from build123d import *
from OCP.BRepFilletAPI import BRepFilletAPI_MakeChamfer

# Parameters (mm, degrees)
EXTRUDE_1_DEPTH     = 1
EXTRUDE_2_DEPTH     = 1
SKETCH_3_W          = 1.5
SKETCH_3_H          = 8
EXTRUDE_3_DEPTH     = 4.5
SKETCH_4_W          = 3
SKETCH_4_H          = 1.3
EXTRUDE_4_DEPTH     = 6
FILLET_1_R          = 1
CHAMFER_1_SIZE      = 0.3
SKETCH_5_W          = 5
SKETCH_5_H          = 2
CUT_EXTRUDE_1_DEPTH = 1
SKETCH_6_W          = 4
SKETCH_6_H          = 1
EXTRUDE_5_DEPTH     = 2.3
SKETCH_7_W          = 1.15
SKETCH_7_H          = 4
EXTRUDE_6_DEPTH     = 1
CUT_EXTRUDE_2_REACH = 20.465
SKETCH_10_W         = 4
SKETCH_10_H         = 1.5
FILLET_2_R          = 0.75
SKETCH_11_W         = 1.15
SKETCH_11_H         = 4
EXTRUDE_7_DEPTH     = 1
CHAMFER_2_SIZE      = 1.2
CHAMFER_2_SIZE2     = 1.043144085


with BuildPart() as part:
    # 草图1 → 凸台-拉伸1 (new body)
    with BuildSketch(Plane(origin=(0, 0, 0), x_dir=(0, 0, -1), z_dir=(1, 0, 0))):
        with BuildLine():
            Line((-8.62016793, -6.710374314), (-8.62016793, 4.289625686))
            ThreePointArc((-8.62016793, 4.289625686), (-8.327274711, 4.996732467), (-7.62016793, 5.289625686))
            Line((-7.62016793, 5.289625686), (12.37983207, 5.289625686))
            ThreePointArc((12.37983207, 5.289625686), (13.086938851, 4.996732467), (13.37983207, 4.289625686))
            Line((13.37983207, 4.289625686), (13.37983207, -6.710374314))
            ThreePointArc((13.37983207, -6.710374314), (13.086938851, -7.417481096), (12.37983207, -7.710374314))
            Line((12.37983207, -7.710374314), (-7.62016793, -7.710374314))
            ThreePointArc((-7.62016793, -7.710374314), (-8.327274711, -7.417481096), (-8.62016793, -6.710374314))
        make_face()
    extrude(amount=EXTRUDE_1_DEPTH)

    # 草图2 → 凸台-拉伸2 (add)
    with BuildSketch(Plane.ZY):
        with BuildLine():
            Line((9.62016793, -6.810374314), (9.62016793, 4.189625686))
            ThreePointArc((9.62016793, 4.189625686), (9.063670815, 5.53312857), (7.72016793, 6.089625686))
            Line((7.72016793, 6.089625686), (-12.27983207, 6.089625686))
            ThreePointArc((-12.27983207, 6.089625686), (-13.623334954, 5.53312857), (-14.17983207, 4.189625686))
            Line((-14.17983207, 4.189625686), (-14.17983207, -6.810374314))
            ThreePointArc((-14.17983207, -6.810374314), (-13.623334954, -8.153877199), (-12.27983207, -8.710374314))
            Line((-12.27983207, -8.710374314), (7.72016793, -8.710374314))
            ThreePointArc((7.72016793, -8.710374314), (9.063670815, -8.153877199), (9.62016793, -6.810374314))
        make_face()
    extrude(amount=EXTRUDE_2_DEPTH)

    # 草图3 → 凸台-拉伸3 (add)
    with BuildSketch(Plane(origin=(1, 0, 0), x_dir=(0, 0, -1), z_dir=(1, 0, 0))):
        with Locations((-6.37016793, -1.310374314)):
            Rectangle(SKETCH_3_W, SKETCH_3_H)
        with Locations((10.92983207, -1.310374314)):
            Rectangle(SKETCH_3_W, SKETCH_3_H)
    extrude(amount=EXTRUDE_3_DEPTH)

    # 草图4 → 凸台-拉伸4 (add)
    with BuildSketch(Plane(origin=(1, 0, 0), x_dir=(0, 0, -1), z_dir=(1, 0, 0))):
        with Locations((-5.62016793, -1.999635097)):
            Rectangle(SKETCH_4_W, SKETCH_4_H)
        with Locations((10.17983207, -1.999635097)):
            Rectangle(SKETCH_4_W, SKETCH_4_H)
    extrude(amount=EXTRUDE_4_DEPTH)

    # 圆角1
    fillet_1_edges = [part.edges().sort_by_distance(p)[0] for p in [
        (7, -1.999635097, -8.67983207),
        (7, -1.999635097, -11.67983207),
        (5.5, -5.310374314, 6.37016793),
        (5.5, 2.689625686, 6.37016793),
        (5.5, -5.310374314, -10.92983207),
        (5.5, 2.689625686, -10.92983207),
        (7, -1.999635097, 7.12016793),
        (7, -1.999635097, 4.12016793),
    ]]
    fillet(fillet_1_edges, radius=FILLET_1_R)

    # 倒角1
    chamfer_1_edges = [part.edges().sort_by_distance(p)[0] for p in [
        (5.75, -2.649635097, 7.12016793),
        (5.75, -1.349635097, 7.12016793),
        (5.75, -1.349635097, -11.67983207),
        (5.75, -2.649635097, -11.67983207),
        (7, -2.649635097, -10.17983207),
        (7, -1.349635097, -10.17983207),
        (3.5, -2.649635097, -8.67983207),
        (6.707106781, -2.649635097, -11.386938851),
        (6.707106781, -2.649635097, -8.972725289),
        (3.5, -1.349635097, -8.67983207),
        (6.707106781, -1.349635097, -11.386938851),
        (6.707106781, -1.349635097, -8.972725289),
        (7, -2.649635097, 5.62016793),
        (7, -1.349635097, 5.62016793),
        (3.5, -2.649635097, 4.12016793),
        (6.707106781, -2.649635097, 4.413061149),
        (6.707106781, -2.649635097, 6.827274711),
        (3.5, -1.349635097, 4.12016793),
        (6.707106781, -1.349635097, 4.413061149),
        (6.707106781, -1.349635097, 6.827274711),
    ]]
    chamfer(chamfer_1_edges, length=CHAMFER_1_SIZE)

    # 草图5 → 切除-拉伸1 (cut)
    with BuildSketch(Plane(origin=(1, 0, 0), x_dir=(0, 0, -1), z_dir=(1, 0, 0))):
        with Locations((2.27983207, -6.710374314)):
            Rectangle(SKETCH_5_W, SKETCH_5_H)
        with Locations((2.27983207, 4.289625686)):
            Rectangle(SKETCH_5_W, SKETCH_5_H)
    extrude(amount=-CUT_EXTRUDE_1_DEPTH, mode=Mode.SUBTRACT)

    # 草图6 → 凸台-拉伸5 (add)
    with BuildSketch(Plane(origin=(0, 0, 0), x_dir=(0, 0, -1), z_dir=(1, 0, 0))):
        with Locations((2.27983207, -7.210374314)):
            Rectangle(SKETCH_6_W, SKETCH_6_H)
        with Locations((2.27983207, 4.789625686)):
            Rectangle(SKETCH_6_W, SKETCH_6_H)
    extrude(amount=EXTRUDE_5_DEPTH)

    # 草图7 → 凸台-拉伸6 (add)
    with BuildSketch(Plane.XZ.offset(7.710374314)):
        with Locations((1.725, -2.27983207)):
            Rectangle(SKETCH_7_W, SKETCH_7_H)
    extrude(amount=EXTRUDE_6_DEPTH)

    # 草图10 → 切除-拉伸2 (cut, up to next)
    with BuildSketch(Plane.ZY.offset(1), mode=Mode.PRIVATE) as cut_extrude_2_sk1:
        with Locations((-2.27983207, -4.523813103)):
            Rectangle(SKETCH_10_W, SKETCH_10_H)
    cut_extrude_2_tool1 = extrude(cut_extrude_2_sk1.sketch, amount=-CUT_EXTRUDE_2_REACH, mode=Mode.PRIVATE) & part.part
    add(cut_extrude_2_tool1.solids().sort_by_distance((-1, -4.523813, -2.279832))[0], mode=Mode.SUBTRACT)

    # 圆角2
    fillet_2_edges = [part.edges().sort_by_distance(p)[0] for p in [
        (0, -5.273813103, -0.27983207),
        (0, -3.773813103, -0.27983207),
        (0, -3.773813103, -4.27983207),
        (0, -5.273813103, -4.27983207),
    ]]
    fillet(fillet_2_edges, radius=FILLET_2_R - 0.0001)  # a hair under: the kernel refuses the full size

    # 草图11 → 凸台-拉伸7 (add)
    with BuildSketch(Plane(origin=(0, 5.289625686, 0), x_dir=(1, 0, 0), z_dir=(0, 1, 0))):
        with Locations((1.725, 2.27983207)):
            Rectangle(SKETCH_11_W, SKETCH_11_H)
    extrude(amount=EXTRUDE_7_DEPTH)

    # 倒角2: one chamfer whose edges measure the first distance from different faces: ONE call of the kernel's chamfer builder (chamfer() names one face for all edges)
    chamfer_2_edges_1 = [part.edges().sort_by_distance(p)[0] for p in [
        (2.3, -8.710374314, -2.27983207),
    ]]
    chamfer_2_side_1 = [part.faces().sort_by_distance(p)[0] for p in [
        (2.3, -7.710374314, -2.27983207),
    ]]
    chamfer_2_edges_2 = [part.edges().sort_by_distance(p)[0] for p in [
        (2.3, 6.289625686, -2.27983207),
    ]]
    chamfer_2_side_2 = [part.faces().sort_by_distance(p)[0] for p in [
        (2.3, 5.289625686, -2.27983207),
    ]]
    chamfer_2 = BRepFilletAPI_MakeChamfer(part.part.solid().wrapped)
    for e in chamfer_2_edges_1:
        chamfer_2.Add(CHAMFER_2_SIZE, CHAMFER_2_SIZE2, e.wrapped, chamfer_2_side_1[0].wrapped)  # the first distance lies on this face
    for e in chamfer_2_edges_2:
        chamfer_2.Add(CHAMFER_2_SIZE, CHAMFER_2_SIZE2, e.wrapped, chamfer_2_side_2[0].wrapped)  # the first distance lies on this face
    add(Compound.cast(chamfer_2.Shape()), mode=Mode.REPLACE)


solid = part.part
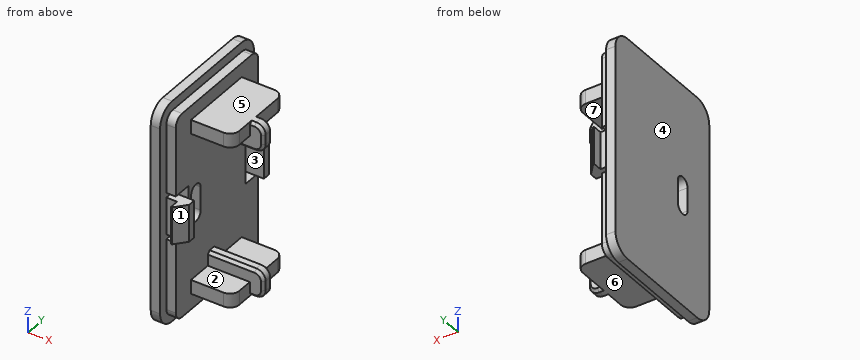
Source: CAD feature listing. Evaluate the final solid. Frame: model axes, mm. Face numbers are marked on the shaded views. A direction names the side the tool comes from. Round coordinates to 2 decimals unless told otherwise and drop trailing zeros. Loops run counter-clockwise (first coordinate to the right, second up) from the corner with the lowest first, then second, coordinate; pieces in that order, holes last. Notation, with made-up numbers: M 56,87 L 69,87 A23 ccw 69,104 Z; hole C 64.25,-30 d11. An arc over 180 degrees is marked long. Return JSON: item names as keys, results as strings. Group by question number.
1. Section query B-B on x = 4. Output: boundary loops of the cut face in (y, z), and give its area (3 significant figures).
2. Section query A-A on z = -2.25. Output: boundary loops of the cut face in (x, y).
3. Mould query, pull axis Y, two halves, no side actions, for the marked faces 1, 2 and 3. Classes: released by +Y, released by -Y, zero draft, split by the parting line, or undercut.
4. Section query D-D on z = 1.25. Output: boundary loops of the cut face in (x, y), and give its area (3 significant figures).
5. Section query C-C on y = -0.5. Output: boundary loops of the cut face in (x, z), and give its area (3 significant figures).
6. Material intervals for line 1 along Z through (x, y) = (3.25, -4.25); line 2 along Y through (x, z) = (4.5, -10); line 3 along X through (y, z) = (5.5, -10.5), sorted ascending. Write a range as from..to.
7. Reachability of the marked faces 4, 5, 6 and 7 from +Z, -Z, +X, -X, +Y, -Y: full face, straight path, thin tool, end or side. Return the list, or none.
8. Pin query (flat end, axial travel): pin 1 (0.8 mm diameter, centred on x = 0.5, z = 5.5, fed in from +Y); pin 2 (1.6 mm diameter, centred on x = 1.5, y = 5.5, fed in from +Z); pin 3 (1.5 mm diameter, centred on x = 4, z = -11, fed in from -Y); pin 4 (1.5 mm diameter, centred on x = 4.5, z = -2, fed in from -Y). Return the tip coordinate at first contact, or that it passes through.
Checks:
{
 "1": {"outline": "M -5.31,-11.68 L 2.69,-11.68 L 2.69,-10.18 L -1.35,-10.18 L -1.35,-8.98 L -1.65,-8.68 L -2.35,-8.68 L -2.65,-8.98 L -2.65,-10.18 L -5.31,-10.18 Z; M -5.31,5.62 L -2.65,5.62 L -2.65,4.42 L -2.35,4.12 L -1.65,4.12 L -1.35,4.42 L -1.35,5.62 L 2.69,5.62 L 2.69,7.12 L -5.31,7.12 Z", "area": "27.7 mm²"},
 "2": {"outline": "M -1,-8.71 L 0,-8.71 L 0,-7.71 L 1.15,-7.71 L 1.15,-8.71 L 1.26,-8.71 L 2.3,-7.51 L 2.3,-6.71 L 0,-6.71 L 0,-5.71 L 1,-5.71 L 1,-5.27 L -1,-5.27 Z; M -1,-3.77 L 1,-3.77 L 1,3.29 L 0,3.29 L 0,4.29 L 2.3,4.29 L 2.3,5.09 L 1.26,6.29 L 1.15,6.29 L 1.15,5.29 L 0,5.29 L 0,6.09 L -1,6.09 Z"},
 "3": {"face 1": "released by -Y", "face 2": "zero draft", "face 3": "undercut"},
 "4": {"outline": "M -1,-8.71 L 0,-8.71 L 0,-7.71 L 1,-7.71 L 1,5.29 L 0,5.29 L 0,6.09 L -1,6.09 Z", "area": "27.8 mm²"},
 "5": {"outline": "M -1,-14.18 L 0,-14.18 L 0,-13.38 L 1,-13.38 L 1,-11.68 L 5.5,-11.68 L 5.5,-10.18 L 1,-10.18 L 1,5.62 L 5.5,5.62 L 5.5,7.12 L 1,7.12 L 1,8.62 L 0,8.62 L 0,9.62 L -1,9.62 Z", "area": "59.3 mm²"},
 "6": {"line 1": "z = -11.68..-10.18, 5.62..7.12", "line 2": "y = -2.65..-1.35", "line 3": "x = -1..0"},
 "7": {"face 4": "+Z, -Z, -X, +Y, -Y", "face 5": "+Z, +X, +Y, -Y", "face 6": "-Z, +X, +Y, -Y", "face 7": "+X, +Y"},
 "8": {"pin 1": "stops at y = 5.29", "pin 2": "stops at z = 8.43", "pin 3": "stops at y = -5.31", "pin 4": "passes through"}
}
